Can you work these out from the model? Positions are in its coordinate system, mm. A direction names the side the tool comes from. Give positions to 0.01 mm unless a question says otherwise; leave off trailing zeros. Loops run counter-clockwise (first coordinate to the right, second up) from the corner with the lowest first, then second, coordinate; pieces in that order, holes last. Notation, with made-up numbers: (84, 70.25) - (95, 70.25) arc R10 ccw to (95, 75.25) - close; hole circle Ø7 at (-27, 11). An arc over 180 degrees is marked (long way). Answer as a JSON object with one key per item and string values. Group by question number.
Item 1: Please list where these lines run through material, in increasing order: L1, parallel to X at y = 2.5, z = -1.75; L2, parallel to Z at x = -8, y = -0.5; L3, parallel to Z at x = 2.5, y = -1.5.
Item 2: Thinking about a two-plate mould opening in Y: for faces 1 (the conical face through (-6.704, -0.047, 0.212)), 2 (the cylindrical face through (2, 0, -2)), 3 (the flat face through (4, 0, 0)), which applies, pulls with the +Y half, pulls with the -Y half, needs draft (parallel to the pull), parting line crosses it, or undercut?
Item 3: Suppose I cut it at A-A on y = -4. Write out the boundary of the cut face in (x, z).
Item 4: Suppose I cut it at B-B on x = -2. Write out the boundary of the cut face in (y, z), and give its area (3 significant figures).
Item 5: Which directions (+Z, -Z, +X, -X, +Y, -Y) give clear straight access to the entire face, cutting with the end or side of a thin tool? Please do faces 4 (the flat face through (-9, 0, -1.25)), 5 (the flat face through (0, 1, -2)), 6 (the cylindrical face through (-8.38, -1.08, -4.88)).
Item 6: Suppose I cut it at D-D on x = 1.75. Write out the boundary of the cut face in (y, z).
Item 7: Suppose I cut it at C-C on z = 3.75. Write out the boundary of the cut face in (x, y).
Item 8: Will these pins go through, and if not, where does the flat tip stop? pin 1 (1.5 mm diameter, centred on x = -6, z = -1.5, fed in from +Y); pin 2 (1.2 mm diameter, centred on y = -0.5, z = 0, fed in from -X); pin 3 (5 mm diameter, centred on x = -8, z = -4, fed in from -Y).
Autodesk Inventor part; units mm, degrees
ref_plane "YZ Plane" through (0, 0, 0) normal (1, 0, 0) x (0, 1, 0)
ref_plane "XZ Plane" through (0, 0, 0) normal (0, 1, 0) x (-1, 0, 0)
ref_plane "XY Plane" through (0, 0, 0) normal (0, 0, 1) x (1, 0, 0)
sketch "Sketch_1" plane through (0, 0, 0) normal (0, 0, 1) x (1, 0, 0)
  line L0 (4, 0) -> (-9.8, 0)
  line L1 (-9.8, 0) -> (-9.8, 5)
  line L2 (-9.8, 5) -> (-7, 5)
  line L3 (-7, 5) -> (-7, 3)
  line L4 (-7, 3) -> (0, 3)
  line L5 (0, 3) -> (0, 2)
  line L6 (0, 2) -> (3.5705, 2)
  line L7 (3.5705, 2) -> (4, 1.5705)
  line L8 (4, 1.5705) -> (4, 0)
  line L9 (4, 0) -> (-9.8, 0)
revolve "Revolution1" add sketch "Sketch_1" angle 360 about axis through (4, 0, 0) along (1, 0, 0)
thread "Thread1"
sketch "Sketch_2" plane through (-9.8, 0, 0) normal (-1, 0, 0) x (0, 1, 0)
  line L0 (-1.4434, 0) -> (-0.7217, -1.25)
  line L1 (-0.7217, -1.25) -> (0.7217, -1.25)
  line L2 (0.7217, -1.25) -> (1.4434, 0)
  line L3 (1.4434, 0) -> (0.7217, 1.25)
  line L4 (0.7217, 1.25) -> (-0.7217, 1.25)
  line L5 (-0.7217, 1.25) -> (-1.4434, 0)
extrude "Extrusion1" cut sketch "Sketch_2" against normal blind 2.5
sketch "Sketch_3" plane through (0, 0, 0) normal (0, 0, 1) x (1, 0, 0)
  line L0 (-6.5783, 0) -> (-7.3, 0)
  line L1 (-7.3, 0) -> (-7.3, 1.25)
  line L2 (-7.3, 1.25) -> (-6.5783, 0)
  line L3 (-6.5783, 0) -> (-7.3, 0)
revolve "Revolution2" cut sketch "Sketch_3" angle 360 about axis through (-6.5783, 0, 0) along (1, 0, 0)
properties part number "DBS4-7-4"
Worked out:
{
 "1": {"L1": "x = -9.8 to -7", "L2": "z = -4.97 to -1.25, 1.25 to 4.97", "L3": "z = -1.32 to 1.32"},
 "2": {"face 1": "undercut", "face 2": "parting line crosses it", "face 3": "needs draft"},
 "3": {"outline": "(-9.8, -3) - (-7, -3) - (-7, 3) - (-9.8, 3) - close"},
 "4": {"outline": "circle Ø6 at (0, 0)", "area": "28.3 mm2"},
 "5": {"face 4": "-X", "face 5": "+X", "face 6": "+X, -X"},
 "6": {"outline": "circle Ø4 at (0, 0)"},
 "7": {"outline": "(-9.8, -3.31) - (-7, -3.31) - (-7, 3.31) - (-9.8, 3.31) - close"},
 "8": {"pin 1": "stops at y = 2.9", "pin 2": "stops at x = -7.21", "pin 3": "stops at y = -4.77"}
}
